from build123d import *

# Parameters (mm, degrees)
SKETCH1_W           = 43.5
SKETCH1_H           = 43.5
BOSS_EXTRUDE2_DEPTH = 2.5
SKETCH3_W           = 43.5
SKETCH3_H           = 43.5
SKETCH3_W_2         = 40.2
SKETCH3_H_2         = 40.2
BOSS_EXTRUDE3_DEPTH = 3
SKETCH4_W           = 10
SKETCH4_H           = 10
CUT_EXTRUDE1_DEPTH  = 5
FILLET1_R           = 2


with BuildPart() as part:
    # Sketch1 → Boss-Extrude2 (new body)
    with BuildSketch(Plane(origin=(0, 0, 0), x_dir=(1, 0, 0), z_dir=(0, 1, 0))):
        Rectangle(SKETCH1_W, SKETCH1_H)
    extrude(amount=BOSS_EXTRUDE2_DEPTH)

    # Sketch3 → Boss-Extrude3 (add)
    with BuildSketch(Plane(origin=(0, 2.5, 0), x_dir=(1, 0, 0), z_dir=(0, 1, 0))):
        Rectangle(SKETCH3_W, SKETCH3_H)
        Rectangle(SKETCH3_W_2, SKETCH3_H_2, mode=Mode.SUBTRACT)
    extrude(amount=BOSS_EXTRUDE3_DEPTH)

    # Sketch4 → Cut-Extrude1 (cut)
    with BuildSketch(Plane(origin=(0, 2.5, 0), x_dir=(1, 0, 0), z_dir=(0, 1, 0))):
        Rectangle(SKETCH4_W, SKETCH4_H)
    extrude(amount=-CUT_EXTRUDE1_DEPTH, mode=Mode.SUBTRACT)

    # Fillet1
    fillet1_edges = [part.edges().sort_by_distance(p)[0] for p in [
        (21.75, 2.75, 21.75),
        (-21.75, 2.75, 21.75),
        (-21.75, 2.75, -21.75),
        (21.75, 2.75, -21.75),
    ]]
    fillet(fillet1_edges, radius=FILLET1_R)


solid = part.part
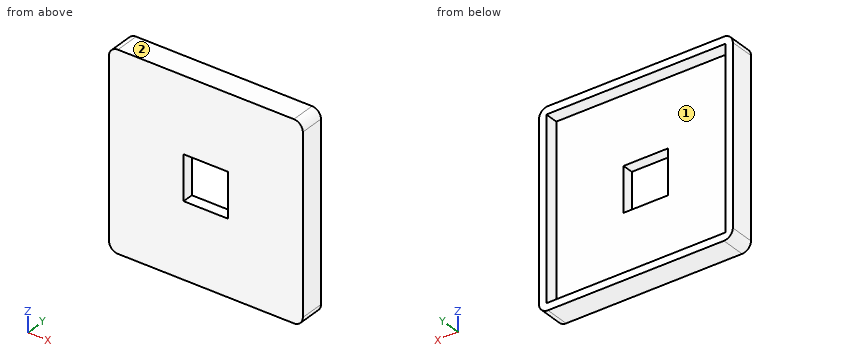
The listing builds one solid part. Answer for the finished solid, in the listing's coordinates (mm). Face numbers are marked on the shaded views. A direction names the side the tool comes from. Round coordinates to 2 decimals unless told otherwise and drop trailing zeros. Write each loop counter-clockwise with the first axis right and the second up, starting at its lowest first coordinate (ties: lowest second). Pieces come first, ordered by that corner, then holes. Notation, with made-up numbers: M 63.5,69 L 105.5,69 A19 cw 105.5,100 Z; hole C 12.5,38 d10. An arc over 180 degrees is marked long. Write each question's results on one line, items separated by ' | '. Start each with the question number.
(1) Find the intervals of material crossed by line 1 (Z direction, x = 17, y = 4.55); line 2 (Y direction, x = 10.5, z = 14), in increasing order.
(2) This flat-tipped pin is pushed along its axis until it touches: P1, Ø1, axis at x = 5, z = -4, coming from the +Y side. Where does it stop, or does it pass through?
(3) The part is cut by section D-D, the plane y = 1.5. Write down the section's boundary in (x, z), and give its area (3 significant figures).
(4) For the marked faces 1 and 2, determine the directions among +Z, -Z, +X, -X, +Y, -Y from which every point of the face is accessible in a straight line to the end or side of a thin tool.
(5) The part is cut by section B-B, the plane y = 4.9. Write down the section's boundary in (x, z), and give its area (3 significant figures).
(6) The part is cut by section C-C, the plane x = -3. Write down the section's boundary in (y, z).
(7) The part is cut by section A-A, the plane z = -0.5. Write down the section's boundary in (x, y).
Worked answers:
1) line 1: z = -21.75 to -20.1, 20.1 to 21.75 | line 2: y = 0 to 2.5
2) P1: stops at y = 2.5
3) outline: M -21.75,-19.75 A2 ccw -19.75,-21.75 L 19.75,-21.75 A2 ccw 21.75,-19.75 L 21.75,19.75 A2 ccw 19.75,21.75 L -19.75,21.75 A2 ccw -21.75,19.75 Z; hole M -5,-5 L 5,-5 L 5,5 L -5,5 Z | area: 1,790 mm²
4) face 1: +Y | face 2: +Z, +X, -X, +Y, -Y
5) outline: M -21.75,-19.75 A2 ccw -19.75,-21.75 L 19.75,-21.75 A2 ccw 21.75,-19.75 L 21.75,19.75 A2 ccw 19.75,21.75 L -19.75,21.75 A2 ccw -21.75,19.75 Z; hole M -20.1,-20.1 L 20.1,-20.1 L 20.1,20.1 L -20.1,20.1 Z | area: 273 mm²
6) outline: M 0,-21.75 L 5.5,-21.75 L 5.5,-20.1 L 2.5,-20.1 L 2.5,-5 L 0,-5 Z; M 0,5 L 2.5,5 L 2.5,20.1 L 5.5,20.1 L 5.5,21.75 L 0,21.75 Z
7) outline: M -21.75,0 L -5,0 L -5,2.5 L -20.1,2.5 L -20.1,5.5 L -21.75,5.5 Z; M 5,0 L 21.75,0 L 21.75,5.5 L 20.1,5.5 L 20.1,2.5 L 5,2.5 Z
